For this review, take the finished solid that the model builds, in its own axes (mm). Face numbers are marked on the shaded views. Round coordinates to 2 decimals unless told otherwise and drop trailing zeros. One line per question, with ' | ' between items.
```python
from build123d import *

# Parameters (mm, degrees)
F0_R     = 301.625
F1_DEPTH = 69.85
F2_R     = 215.9
F3_DEPTH = 32.0625
F3_TAPER = 3
F4_R     = 180
F5_DEPTH = 101.9135
F10_D    = 38.1


with BuildPart() as f1:
    # F0 (on Top) → F1 (new body)
    with BuildSketch(Plane.XY):
        Circle(F0_R)
    extrude(amount=-F1_DEPTH)

    # F2 (on face) → F3 (join)
    with BuildSketch(Plane(origin=(0, 0, -69.85), x_dir=(1, 0, 0), z_dir=(0, 0, -1))):
        Circle(F2_R)
    extrude(amount=F3_DEPTH, taper=F3_TAPER)

    # F4 (on face) → F5 (cut, through all)
    with BuildSketch(Plane(origin=(0, 0, -101.9125), x_dir=(1, 0, 0), z_dir=(0, 0, -1))):
        Circle(F4_R)
    extrude(amount=-F5_DEPTH, mode=Mode.SUBTRACT)

    # F6 (on Front) → F8 (revolve, cut)
    with BuildSketch(Plane.XZ):
        Polygon((209.55, -7.9375), (209.55, 0), (203.596875, 0), (206.9661438537, -7.9375), align=None)
        Polygon((215.503125, 0), (209.55, 0), (209.55, -7.9375), (212.1338561463, -7.9375), align=None)
    revolve(axis=Axis((0, 0, 0), (0, 0, 1)), mode=Mode.SUBTRACT)

    # F10 (through all)
    with Locations(Plane.XY):
        with Locations((263.525, 0), (250.6271684567, 81.4337034427), (213.1962034427, 154.8961086104), (154.8961086104, 213.1962034427), (81.4337034427, 250.6271684567), (0, 263.525), (-81.4337034427, 250.6271684567), (-154.8961086104, 213.1962034427), (-213.1962034427, 154.8961086104), (-250.6271684567, 81.4337034427), (-263.525, 0), (-250.6271684567, -81.4337034427), (-213.1962034427, -154.8961086104), (-154.8961086104, -213.1962034427), (-81.4337034427, -250.6271684567), (0, -263.525), (81.4337034427, -250.6271684567), (154.8961086104, -213.1962034427), (213.1962034427, -154.8961086104), (250.6271684567, -81.4337034427)):
            Hole(F10_D / 2)


solid = f1.part
```
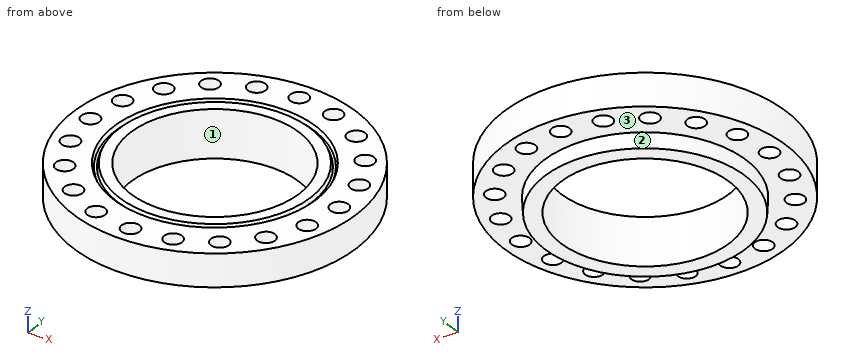
(1) We need section A-A on x = 0. Give the number of separate pieces and of enclosed holes in the cut face, plus the area to 3 significant figures.
Output values:
separate pieces: 4 | enclosed holes: 0 | area: 13,800 mm^2
(2) Mouldability with a two-part tool opening along X and no side actions: class the marked faces 1, 2 and 3 as released by +X, released by -X, zero draft, split by the parting line, or undercut.
Output values:
face 1: undercut | face 2: split by the parting line | face 3: zero draft
(3) For probe 1 along Y at (x, z) = (1, -27.5); probe 2 along X at (y, z) = (252.5, -40.5); probe 3 along X at (y, z) = (-12, -65.5), list the stretches that pass through material, from the lowest coordinate up. Write a range as [from, to].
Output values:
probe 1: [-301.62, -282.55], [-244.5, -180], [180, 244.5], [282.55, 301.62] | probe 2: [-164.99, -100.39], [-62.48, -15.54], [15.54, 62.48], [100.39, 164.99] | probe 3: [-301.39, -278.32], [-248.73, -179.6], [179.6, 248.73], [278.32, 301.39]
(4) Insertion check: pin 1 (1 mm diameter, centred on x = 141, z = -83.5, fed in from +Y); pin 2 (4 mm diameter, centred on x = 170, z = -67, fed in from +Y); pin 3 (3 mm diameter, centred on y = 224.5, z = -63, fed in from +X); pin 4 (6 mm diameter, centred on x = 188.5, y = -15.5, fed in from +Z). Each pin has a flat end and moves straight along its axis. Give the tip position at first contact, or say it passes through.
Output values:
pin 1: y = 162.99 | pin 2: y = 250.51 | pin 3: x = 203.1 | pin 4: z = 0
